For this review, take the finished solid that the model builds, in its own axes (mm). Face numbers are marked on the shaded views. A direction names the side the tool comes from. Give positions to 0.01 mm unless a question says otherwise; leave off trailing zeros. Order: outer loops, then holes, each group sorted by start corner. A loop starts at its lowest first (then second) coordinate and runs counter-clockwise, first axis right, second up.
Item 1: The part is to be moulded in two halves that separate along X. For the marked faces 4, 5, 6 and 7, say which applies: released by +X, released by -X, zero draft, split by the parting line, or undercut.
Item 2: Machinability: for the marked faces 1, 2 and 3, which of the approach directions +Z, -Z, +X, -X, +Y, -Y give a long, thin tool a straight path to every point of the face, cutting with its end or side? Answer none if there is none.
Item 3: Consider section B-B (y = -0.75). Give the boundary of the cut face in (x, z).
Item 4: Consider section A-A (x = 0). Give the boundary of the cut face in (y, z).
Item 5: For probe 1 along X at (y, z) = (-5.5, 1.95); probe 2 along Y at (x, z) = (0, 1.1); probe 3 along X at (y, z) = (-4.25, 2.4), list the stretches that pass through material, from the lowest coordinate up.
```python
from build123d import *

# Parameters (mm, degrees)
RESSALTO_EXTRUS_O1_DEPTH = 2.5
ESBO_O2_R                = 1.65
CORTE_EXTRUS_O1_DEPTH    = 11.891664024


with BuildPart() as part:
    # Esboço1 → Ressalto-extrusão1 (new body)
    with BuildSketch(Plane.XY):
        with BuildLine():
            Line((2.274601503, 6.165929395), (2.745743779, 6.813655149))
            ThreePointArc((2.745743779, 6.813655149), (2.854880588, 6.888968105), (2.987139863, 6.879461857))
            ThreePointArc((2.987139863, 6.879461857), (3.480600792, 6.643449264), (3.955547671, 6.372098761))
            ThreePointArc((3.955547671, 6.372098761), (4.038558016, 6.269040995), (4.03904852, 6.136710424))
            Line((4.03904852, 6.136710424), (3.776369648, 5.378426201))
            ThreePointArc((3.776369648, 5.378426201), (3.775484994, 5.315635516), (3.812211303, 5.264697995))
            ThreePointArc((3.812211303, 5.264697995), (4.307643395, 4.867669707), (4.76197859, 4.424201613))
            ThreePointArc((4.76197859, 4.424201613), (4.817162567, 4.393913756), (4.879509874, 4.402599311))
            Line((4.879509874, 4.402599311), (5.597698808, 4.75718125))
            ThreePointArc((5.597698808, 4.75718125), (5.729334329, 4.773149156), (5.842026327, 4.703267842))
            ThreePointArc((5.842026327, 4.703267842), (6.16928376, 4.264966341), (6.463725469, 3.803978583))
            ThreePointArc((6.463725469, 3.803978583), (6.489334147, 3.674148632), (6.428271384, 3.556747783))
            Line((6.428271384, 3.556747783), (5.843288544, 3.007393407))
            ThreePointArc((5.843288544, 3.007393407), (5.813324936, 2.952206135), (5.822172622, 2.890035634))
            ThreePointArc((5.822172622, 2.890035634), (6.076347708, 2.308245771), (6.272551644, 1.704434182))
            ThreePointArc((6.272551644, 1.704434182), (6.30733916, 1.651970343), (6.366581337, 1.630686782))
            Line((6.366581337, 1.630686782), (7.1672885, 1.610894457))
            ThreePointArc((7.1672885, 1.610894457), (7.291266621, 1.563859258), (7.358574964, 1.449611845))
            ThreePointArc((7.358574964, 1.449611845), (7.444658166, 0.909431028), (7.491141658, 0.364412755))
            ThreePointArc((7.491141658, 0.364412755), (7.45348203, 0.237553096), (7.344854743, 0.161977088))
            Line((7.344854743, 0.161977088), (6.571580455, -0.052596974))
            ThreePointArc((6.571580455, -0.052596974), (6.519402194, -0.087538093), (6.498344357, -0.146699062))
            ThreePointArc((6.498344357, -0.146699062), (6.453033988, -0.779969455), (6.346158708, -1.40579858))
            ThreePointArc((6.346158708, -1.40579858), (6.352580363, -1.468419567), (6.395145742, -1.514796437))
            Line((6.395145742, -1.514796437), (7.094938772, -1.904428843))
            ThreePointArc((7.094938772, -1.904428843), (7.182857599, -2.003691949), (7.189362757, -2.136132756))
            ThreePointArc((7.189362757, -2.136132756), (7.014551104, -2.654443974), (6.802427572, -3.158635644))
            ThreePointArc((6.802427572, -3.158635644), (6.710127004, -3.253462991), (6.578820396, -3.269900606))
            Line((6.578820396, -3.269900606), (5.794402479, -3.100538022))
            ThreePointArc((5.794402479, -3.100538022), (5.731962976, -3.1072284), (5.685823714, -3.149826772))
            ThreePointArc((5.685823714, -3.149826772), (5.351407949, -3.689503078), (4.965937293, -4.193979829))
            ThreePointArc((4.965937293, -4.193979829), (4.942521962, -4.25241225), (4.958659327, -4.313258047))
            Line((4.958659327, -4.313258047), (5.397224074, -4.983470446))
            ThreePointArc((5.397224074, -4.983470446), (5.428942465, -5.112221478), (5.373154184, -5.232515085))
            ThreePointArc((5.373154184, -5.232515085), (4.977494919, -5.610217851), (4.555359307, -5.958078683))
            ThreePointArc((4.555359307, -5.958078683), (4.429562747, -5.999149916), (4.305657579, -5.952683478))
            Line((4.305657579, -5.952683478), (3.689796725, -5.438183174))
            ThreePointArc((3.689796725, -5.438183174), (3.631400117, -5.415090125), (3.57074938, -5.431367127))
            ThreePointArc((3.57074938, -5.431367127), (3.023838841, -5.753816009), (2.448079489, -6.021370842))
            ThreePointArc((2.448079489, -6.021370842), (2.400191343, -6.062228535), (2.386203819, -6.12360422))
            Line((2.386203819, -6.12360422), (2.463070385, -6.920859027))
            ThreePointArc((2.463070385, -6.920859027), (2.431322037, -7.049602675), (2.32602074, -7.130191268))
            ThreePointArc((2.32602074, -7.130191268), (1.800154633, -7.280758429), (1.264713122, -7.392597698))
            ThreePointArc((1.264713122, -7.392597698), (1.134239047, -7.370503893), (1.0461205, -7.271778302))
            Line((1.0461205, -7.271778302), (0.739903009, -6.530006099))
            ThreePointArc((0.739903009, -6.530006099), (0.698927256, -6.482419963), (0.637659395, -6.468646728))
            ThreePointArc((0.637659395, -6.468646728), (0.003544695, -6.499999033), (-0.630603823, -6.46933836))
            ThreePointArc((-0.630603823, -6.46933836), (-0.691994187, -6.483261319), (-0.732902228, -6.531106463))
            Line((-0.732902228, -6.531106463), (-1.035343047, -7.27276221))
            ThreePointArc((-1.035343047, -7.27276221), (-1.123284969, -7.372004856), (-1.253976023, -7.394426559))
            ThreePointArc((-1.253976023, -7.394426559), (-1.789579385, -7.283364993), (-2.315663597, -7.133561671))
            ThreePointArc((-2.315663597, -7.133561671), (-2.42092515, -7.053364252), (-2.453070179, -6.924996352))
            Line((-2.453070179, -6.924996352), (-2.37949357, -6.125883321))
            ThreePointArc((-2.37949357, -6.125883321), (-2.393661418, -6.064705508), (-2.441510673, -6.02403732))
            ThreePointArc((-2.441510673, -6.02403732), (-3.017561497, -5.757110613), (-3.564823398, -5.435258424))
            ThreePointArc((-3.564823398, -5.435258424), (-3.625652188, -5.419057068), (-3.684109206, -5.442410924))
            Line((-3.684109206, -5.442410924), (-4.296571863, -5.958563217))
            ThreePointArc((-4.296571863, -5.958563217), (-4.420560925, -6.005569567), (-4.546701991, -5.964687838))
            ThreePointArc((-4.546701991, -5.964687838), (-4.969342333, -5.617440412), (-5.365549693, -5.240312634))
            ThreePointArc((-5.365549693, -5.240312634), (-5.42148457, -5.120383863), (-5.390292042, -4.991781193))
            Line((-5.390292042, -4.991781193), (-4.953776848, -4.318394499))
            ThreePointArc((-4.953776848, -4.318394499), (-4.937891107, -4.257640109), (-4.961360069, -4.199393559))
            ThreePointArc((-4.961360069, -4.199393559), (-5.347380717, -3.695337532), (-5.682384894, -3.156026285))
            ThreePointArc((-5.682384894, -3.156026285), (-5.728716967, -3.113412148), (-5.791331164, -3.10692463))
            Line((-5.791331164, -3.10692463), (-6.573507845, -3.2793292))
            ThreePointArc((-6.573507845, -3.2793292), (-6.705139647, -3.263330665), (-6.797833327, -3.168511015))
            ThreePointArc((-6.797833327, -3.168511015), (-7.010688839, -2.664627929), (-7.186253016, -2.146571125))
            ThreePointArc((-7.186253016, -2.146571125), (-7.180047212, -2.014385238), (-7.092662959, -1.91500912))
            Line((-7.092662959, -1.91500912), (-6.39320955, -1.52161354))
            ThreePointArc((-6.39320955, -1.52161354), (-6.350909451, -1.475200671), (-6.344621664, -1.412719342))
            ThreePointArc((-6.344621664, -1.412719342), (-6.452179456, -0.787007155), (-6.498180491, -0.153786559))
            ThreePointArc((-6.498180491, -0.153786559), (-6.519401727, -0.094522027), (-6.571828945, -0.059679346))
            Line((-6.571828945, -0.059679346), (-7.344532399, 0.151159617))
            ThreePointArc((-7.344532399, 0.151159617), (-7.453651682, 0.226497964), (-7.491662971, 0.353533496))
            ThreePointArc((-7.491662971, 0.353533496), (-7.44597102, 0.898618699), (-7.360672377, 1.43892396))
            ThreePointArc((-7.360672377, 1.43892396), (-7.293747566, 1.553084768), (-7.170190267, 1.600468464))
            Line((-7.170190267, 1.600468464), (-6.36803499, 1.623750744))
            ThreePointArc((-6.36803499, 1.623750744), (-6.309010977, 1.645189462), (-6.274406897, 1.697591851))
            ThreePointArc((-6.274406897, 1.697591851), (-6.07886164, 2.301617076), (-5.825321249, 2.883683815))
            ThreePointArc((-5.825321249, 2.883683815), (-5.816570119, 2.946021952), (-5.846799914, 3.001237757))
            Line((-5.846799914, 3.001237757), (-6.433013092, 3.547019587))
            ThreePointArc((-6.433013092, 3.547019587), (-6.494621942, 3.66443864), (-6.469242912, 3.794587744))
            ThreePointArc((-6.469242912, 3.794587744), (-6.175470974, 4.256002613), (-5.848850402, 4.694778906))
            ThreePointArc((-5.848850402, 4.694778906), (-5.736538252, 4.764761771), (-5.605113396, 4.749298011))
            Line((-5.605113396, 4.749298011), (-4.884020357, 4.3971333))
            ThreePointArc((-4.884020357, 4.3971333), (-4.82179412, 4.388686517), (-4.766801124, 4.419005209))
            ThreePointArc((-4.766801124, 4.419005209), (-4.31294988, 4.862968572), (-3.817951111, 5.260536979))
            ThreePointArc((-3.817951111, 5.260536979), (-3.781232394, 5.311667805), (-3.782339484, 5.374607458))
            Line((-3.782339484, 5.374607458), (-4.047768011, 6.130300117))
            ThreePointArc((-4.047768011, 6.130300117), (-4.047752584, 6.262900585), (-3.964797265, 6.36634767))
            ThreePointArc((-3.964797265, 6.36634767), (-3.490244951, 6.638387619), (-2.997127286, 6.875116583))
            ThreePointArc((-2.997127286, 6.875116583), (-2.865157157, 6.884889274), (-2.755972594, 6.810120618))
            Line((-2.755972594, 6.810120618), (-2.28113552, 6.163185609))
            ThreePointArc((-2.28113552, 6.163185609), (-2.229962339, 6.126788379), (-2.167178661, 6.128077729))
            ThreePointArc((-2.167178661, 6.128077729), (-1.558993279, 6.310272574), (-0.935934386, 6.432264518))
            ThreePointArc((-0.935934386, 6.432264518), (-0.879659896, 6.460474577), (-0.851390661, 6.516719362))
            Line((-0.851390661, 6.516719362), (-0.73522806, 7.309202767))
            ThreePointArc((-0.73522806, 7.309202767), (-0.67359189, 7.426607482), (-0.552064345, 7.479654067))
            ThreePointArc((-0.552064345, 7.479654067), (-0.005445871, 7.499998023), (0.541201571, 7.480447905))
            ThreePointArc((0.541201571, 7.480447905), (0.662596914, 7.427771616), (0.724528315, 7.310826663))
            Line((0.724528315, 7.310826663), (0.844329975, 6.517326369))
            ThreePointArc((0.844329975, 6.517326369), (0.87272694, 6.46131686), (0.928918317, 6.433281492))
            ThreePointArc((0.928918317, 6.433281492), (1.552109894, 6.311969176), (2.160493629, 6.130437772))
            ThreePointArc((2.160493629, 6.130437772), (2.223432083, 6.12926448), (2.274601503, 6.165929395))
        make_face()
    extrude(amount=RESSALTO_EXTRUS_O1_DEPTH)

    # Esboço2 → Corte-extrusão1 (cut, through all)
    with BuildSketch(Plane.XY.offset(2.5)):
        Circle(ESBO_O2_R)
    extrude(amount=-CORTE_EXTRUS_O1_DEPTH, mode=Mode.SUBTRACT)


solid = part.part
```
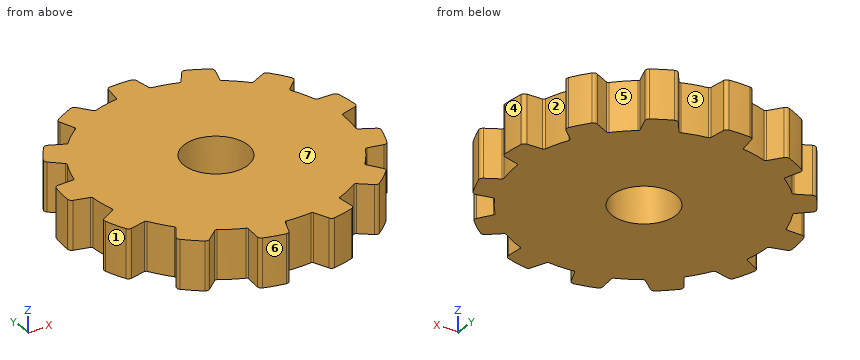
Resolved:
1. face 4: released by +X
1. face 5: undercut
1. face 6: released by -X
1. face 7: zero draft
2. face 1: +Z, -Z, -X, -Y
2. face 2: +Z, -Z, +X
2. face 3: +Z, -Z, +Y
3. outline: (-6.46, 0) - (-1.47, 0) - (-1.47, 2.5) - (-6.46, 2.5) - close; (1.47, 0) - (6.46, 0) - (6.46, 2.5) - (1.47, 2.5) - close
4. outline: (-6.5, 0) - (-1.65, 0) - (-1.65, 2.5) - (-6.5, 2.5) - close; (1.65, 0) - (7.5, 0) - (7.5, 2.5) - (1.65, 2.5) - close
5. probe 1: x = -5.1 to -3.75, -3.46 to 3.46, 3.76 to 5.1
5. probe 2: y = -6.5 to -1.65, 1.65 to 7.5
5. probe 3: x = -4.94 to 4.94
